Can you work these out from the model? Positions are in its coordinate system, mm. Face numbers are marked on the shaded views. Give positions to 0.01 mm unless a question says otherwise; leave off trailing zeros. Order: outer loops, then holes, each group sorted by start corner. A loop starts at its lowest first (then second) coordinate and runs counter-clockwise, first axis right, second up.
Item 1: I want a section at D-D, the plane z = -8. Write out the boundary of the cut face in (x, y), then the cut area to 3 significant figures.
Item 2: I want a section at A-A, the plane z = 0. Write out the boundary of the cut face in (x, y), then the cut area to 3 significant figures.
Item 3: If I drill on line 1 along X through (y, z) = (4, 0); line 2 along Z through (x, y) = (-92, 5.25); line 3 along X through (y, z) = (4.5, -1), over which ranges is the centre line in solid material (lowest first)?
Item 4: I want a section at C-C, the plane y = 2. Write out the boundary of the cut face in (x, z) (3 decimals), then the cut area to 3 significant figures.
Item 5: I'm going to push a flat-ended pin straight in: pin 1 Ø8.5 at (x, z) = (-38.227, 0) entering from +Y. Where does the tip first touch, or does it pass through?
Item 6: I want a section at B-B, the plane x = 38.5. Write out the boundary of the cut face in (y, z).
Item 7: If we mould it in two halves opening along Z, with no side actions, what happens to the marked faces 1 and 2? For each: +Z half, -Z half, draft (parallel to the pull), parting line (faces both ways), or undercut.
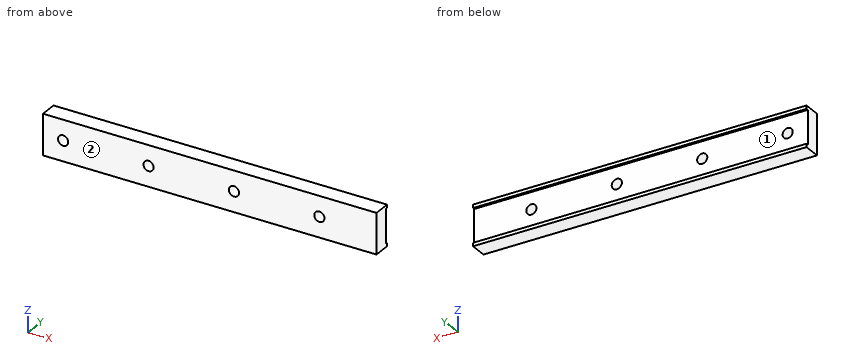
```python
from build123d import *

# Parameters (mm, degrees)
SKETCH1_W           = 208.28
SKETCH1_H           = 25.3746
SKETCH1_R           = 3.175
BOSS_EXTRUDE1_DEPTH = 9.398
SKETCH2_W           = 208.28
SKETCH2_H           = 2.0828
BOSS_EXTRUDE2_DEPTH = 1.27


with BuildPart() as part:
    # Sketch1 → Boss-Extrude1 (new body)
    with BuildSketch(Plane(origin=(0, 0, 0), x_dir=(1, 0, 0), z_dir=(0, 1, 0))):
        Rectangle(SKETCH1_W, SKETCH1_H)
        with Locations(Location((-91.567, 0, 0), (0, 0, 270))):
            Circle(SKETCH1_R, mode=Mode.SUBTRACT)
        with Locations(Location((-38.227, 0, 0), (0, 0, 270))):
            Circle(SKETCH1_R, mode=Mode.SUBTRACT)
        with Locations(Location((15.113, 0, 0), (0, 0, 270))):
            Circle(SKETCH1_R, mode=Mode.SUBTRACT)
        with Locations(Location((68.453, 0, 0), (0, 0, 270))):
            Circle(SKETCH1_R, mode=Mode.SUBTRACT)
    extrude(amount=BOSS_EXTRUDE1_DEPTH)

    # Sketch2 → Boss-Extrude2 (add)
    with BuildSketch(Plane(origin=(0, 9.398, 0), x_dir=(1, 0, 0), z_dir=(0, 1, 0))):
        with Locations((0, 11.6459)):
            Rectangle(SKETCH2_W, SKETCH2_H)
        with Locations((0, -11.6459)):
            Rectangle(SKETCH2_W, SKETCH2_H)
    extrude(amount=BOSS_EXTRUDE2_DEPTH)


solid = part.part
```
Results list:
1. outline: (-104.14, 0) - (104.14, 0) - (104.14, 9.4) - (-104.14, 9.4) - close
1. area: 1,960 mm2
2. outline: (-104.14, 0) - (-94.74, 0) - (-94.74, 9.4) - (-104.14, 9.4) - close; (-88.39, 0) - (-41.4, 0) - (-41.4, 9.4) - (-88.39, 9.4) - close; (-35.05, 0) - (11.94, 0) - (11.94, 9.4) - (-35.05, 9.4) - close; (18.29, 0) - (65.28, 0) - (65.28, 9.4) - (18.29, 9.4) - close; (71.63, 0) - (104.14, 0) - (104.14, 9.4) - (71.63, 9.4) - close
2. area: 1,720 mm2
3. line 1: x = -104.14 to -94.74, -88.39 to -41.4, -35.05 to 11.94, 18.29 to 65.28, 71.63 to 104.14
3. line 2: z = -12.69 to -3.15, 3.15 to 12.69
3. line 3: x = -104.14 to -94.58, -88.55 to -41.24, -35.21 to 12.1, 18.13 to 65.44, 71.47 to 104.14
4. outline: (-104.14, -12.687) - (104.14, -12.687) - (104.14, 12.687) - (-104.14, 12.687) - close; hole circle Ø6.35 at (-91.567, 0); hole circle Ø6.35 at (-38.227, 0); hole circle Ø6.35 at (15.113, 0); hole circle Ø6.35 at (68.453, 0)
4. area: 5,160 mm2
5. pin 1: stops at y = 9.4
6. outline: (0, -12.69) - (10.67, -12.69) - (10.67, -10.6) - (9.4, -10.6) - (9.4, 10.6) - (10.67, 10.6) - (10.67, 12.69) - (0, 12.69) - close
7. face 1: undercut
7. face 2: draft
